Can you work these out from the model? Positions are in its coordinate system, mm. Face numbers are marked on the shaded views. A direction names the side the tool comes from. Give positions to 0.01 mm unless a question says otherwise; leave off trailing zeros. Order: outer loops, then holes, each group sorted by start corner. A loop starts at its lowest first (then second) coordinate and runs counter-clockwise, first axis right, second up. Notation, with made-up numbers: M -30.5,66 L -18.5,66 A24 cw -18.5,84 Z; hole C -36,46.5 d6. An arc over 180 degrees is marked long. Answer as a JSON object with one key per item and string values.
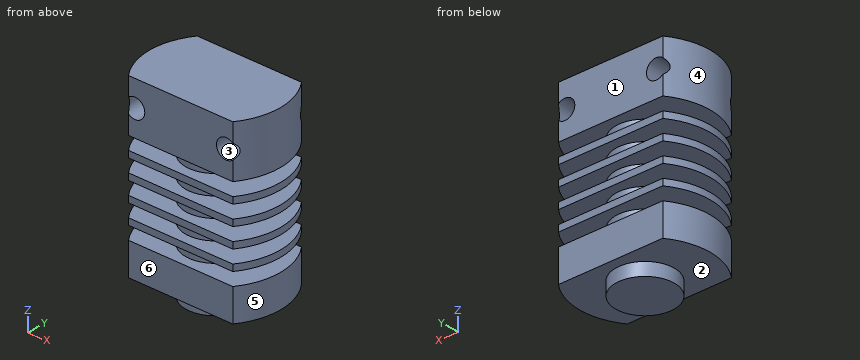
```python
from build123d import *

# Parameters (mm, degrees)
F1_DEPTH      = 27
F2_W          = 30
F2_H          = 2
F3_DEPTH      = 6
F4_R          = 4.5
F5_DEPTH      = 27
F5_DEPTH_BACK = 2
F6_R          = 1.5
F7_DEPTH      = 6


with BuildPart() as f1:
    # F0 (on Top) → F1 (new body)
    with BuildSketch(Plane.XY):
        with BuildLine():
            Line((-8, -6), (8, -6))
            ThreePointArc((8, -6), (10, 0), (8, 6))
            Line((8, 6), (-8, 6))
            ThreePointArc((-8, 6), (-10, 0), (-8, -6))
        make_face()
    extrude(amount=F1_DEPTH)

    # F2 (on Front) → F3 (cut, symmetric)
    with BuildSketch(Plane.XZ):
        with Locations((0, 6)):
            Rectangle(F2_W, F2_H)
        with Locations((0, 9)):
            Rectangle(F2_W, F2_H)
        with Locations((0, 12)):
            Rectangle(F2_W, F2_H)
        with Locations((0, 15)):
            Rectangle(F2_W, F2_H)
        with Locations((0, 18)):
            Rectangle(F2_W, F2_H)
    extrude(amount=F3_DEPTH, both=True, mode=Mode.SUBTRACT)

    # F4 (on Top) → F5 (join, two sides)
    with BuildSketch(Plane.XY) as f5_sk:
        Circle(F4_R)
    extrude(amount=F5_DEPTH)
    extrude(f5_sk.sketch, amount=-F5_DEPTH_BACK)

    # F6 (on Front) → F7 (cut, symmetric)
    with BuildSketch(Plane.XZ):
        with Locations((-7, 23)):
            Circle(F6_R)
        with Locations((7, 23)):
            Circle(F6_R)
    extrude(amount=F7_DEPTH, both=True, mode=Mode.SUBTRACT)


solid = f1.part
```
1) For the marked faces 1 and 2, which set-ups out of +Z, -Z, +X, -X, +Y, -Y let a thin tool reach every point of the face, with its end or its side?
Results found:
{"face 1": "+Z, -Z, +X, -X, +Y", "face 2": "-Z"}
2) I need wall thicknesses on L1, parallel to Z at x = 3.25, y = -4.75; L2, parallel to X at y = -1.25, z = 4; L3, parallel to X at y = -4, z = 10.5. Which ranges of each line are inside material? Lowest first, please.
Results found:
{"L1": "z = 0 to 5, 7 to 8, 10 to 11, 13 to 14, 16 to 17, 19 to 27", "L2": "x = -9.92 to 9.92", "L3": "x = -9.17 to 9.17"}
3) I want a section at D-D on z = 19.5. Write out the boundary of the cut face in (x, y).
Results found:
{"outline": "M -8,-6 L 8,-6 A10 ccw 8,6 L -8,6 A10 ccw Z"}
4) Thinking about a two-plate mould opening in X: for the marked faces 3, 4, 5 and 6, which applies, pulls with the +X half, pulls with the -X half, needs draft (parallel to the pull), parting line crosses it, or undercut?
Results found:
{"face 3": "undercut", "face 4": "pulls with the -X half", "face 5": "pulls with the +X half", "face 6": "needs draft"}
5) I want a section at C-C on y = -1. Count the separate pieces of the cut face and the enclosed holes in it, and give its area (3 significant figures).
Results found:
{"separate pieces": "1", "enclosed holes": "2", "area": "429 mm²"}
6) I'm going to push a flat-ended pin straight in: pin 1 Ø1 at (x, y) = (6, 1.5) entering from -Z. Where does the tip first touch, or does it pass through?
Results found:
{"pin 1": "stops at z = 0"}
7) I want a section at A-A on x = 7. Write out the boundary of the cut face in (y, z), and give its area (3 significant figures).
Results found:
{"outline": "M -6,0 L 6,0 L 6,5 L -6,5 Z; M -6,7 L 6,7 L 6,8 L -6,8 Z; M -6,10 L 6,10 L 6,11 L -6,11 Z; M -6,13 L 6,13 L 6,14 L -6,14 Z; M -6,16 L 6,16 L 6,17 L -6,17 Z; M -6,19 L 6,19 L 6,21.5 L -6,21.5 Z; M -6,24.5 L 6,24.5 L 6,27 L -6,27 Z", "area": "168 mm²"}
8) I want a section at B-B on z = 23. Write out the boundary of the cut face in (x, y).
Results found:
{"outline": "M -8.5,-5.27 L -8.5,5.27 A10 ccw Z; M -5.5,-6 L 5.5,-6 L 5.5,6 L -5.5,6 Z; M 8.5,-5.27 A10 ccw 8.5,5.27 Z"}
